Verification items for the finished model (mm, model axes). Round coordinates to 2 decimals unless told otherwise and drop trailing zeros. Write each loop counter-clockwise with the first axis right and the second up, starting at its lowest first coordinate (ties: lowest second). Pieces come first, ordered by that corner, then holes. Notation, with made-up numbers: (-28, 59) - (9, 59) arc R24 cw to (9, 92) - close; hole circle Ø4 at (37.25, 56.25). An arc over 180 degrees is marked (long way). Answer as a JSON object with one key per item and string values.
```python
from build123d import *

# Parameters (mm, degrees)
CROQUIS3_R              = 6.5
CROQUIS3_R_2            = 4.5
SALIENTE_EXTRUIR1_DEPTH = 7.5
CORTAR_EXTRUIR1_DEPTH   = 7.5


with BuildPart() as part:
    # Croquis2 → Revolución1 (revolve)
    with BuildSketch(Plane.XY):
        Polygon((-4.5, 0), (-8, 7.5), (-10, 7.5), (-6.5, 0), align=None)
    revolve(axis=Axis((0, 7.5, 0), (0, -1, 0)))

    # Croquis3 → Saliente-Extruir1 (add)
    with BuildSketch(Plane.XZ):
        Circle(CROQUIS3_R)
        Circle(CROQUIS3_R_2, mode=Mode.SUBTRACT)
    extrude(amount=SALIENTE_EXTRUIR1_DEPTH)

    # Croquis4 → Cortar-Extruir1 (cut)
    with BuildSketch(Plane(origin=(0, 7.5, 0), x_dir=(1, 0, 0), z_dir=(0, 1, 0))):
        Polygon((-9.027753826, 8), (9.027753826, 8), (9.027753826, 15.356589522), (-9.467057566, 15.356589522), align=None)
    extrude(amount=-CORTAR_EXTRUIR1_DEPTH, mode=Mode.SUBTRACT)


solid = part.part
```
1. Material ranges on probe 1 along X at (y, z) = (-5.25, 0); probe 2 along Z at (x, y) = (2, 3.5), recorded low to high. Write a range as from..to.
Completed:
{"probe 1": "x = -6.5..-4.5, 4.5..6.5", "probe 2": "z = -7.88..-5.8, 5.8..7.88"}
2. Mould release check, pull along Z, two halves, no side actions. Record for faces 1 (the face through (0, 6, -8)), 2 (the face through (1.107, 1.302, 4.986)), 3 (the face through (-5.158, -3.698, -3.955)), 4 (the face through (-4.42, -7.5, 1.54)): released by +Z, released by -Z, zero draft, split by the parting line, or undercut.
Completed:
{"face 1": "released by -Z", "face 2": "undercut", "face 3": "split by the parting line", "face 4": "zero draft"}
3. Go/stop test with flat-tipped pins: pin 1 (3 mm diameter, centred on x = 3.5, y = -0.5, fed in from -Z); pin 2 (6 mm diameter, centred on y = 3, z = 8, fed in from -X); pin 3 (3 mm diameter, centred on x = 1.5, z = -1, fed in from -Y); pin 4 (2 mm diameter, centred on x = -5, z = 7, fed in from -Y). Record where each tip stops, or that it passes through.
Completed:
{"pin 1": "stops at z = -6.31", "pin 2": "stops at x = -6.71", "pin 3": "passes through", "pin 4": "stops at y = 2.36"}
4. Cross-section at A-A (z = 0). Record the boundary of the cut face in (x, y), plus the area to 3 significant figures.
Completed:
{"outline": "(-10, 7.5) - (-6.5, 0) - (-6.5, -7.5) - (-4.5, -7.5) - (-4.5, 0) - (-8, 7.5) - close; (4.5, -7.5) - (6.5, -7.5) - (6.5, 0) - (10, 7.5) - (8, 7.5) - (4.5, 0) - close", "area": "60.0 mm^2"}
5. Cross-section at C-C (y = 2). Record the boundary of the cut face in (x, z), plus the area to 3 significant figures.
Completed:
{"outline": "circle Ø14.87 at (0, 0); hole circle Ø10.87 at (0, 0)", "area": "80.8 mm^2"}
6. Cross-section at B-B (y = -6.5). Record the boundary of the cut face in (x, z).
Completed:
{"outline": "circle Ø13 at (0, 0); hole circle Ø9 at (0, 0)"}
